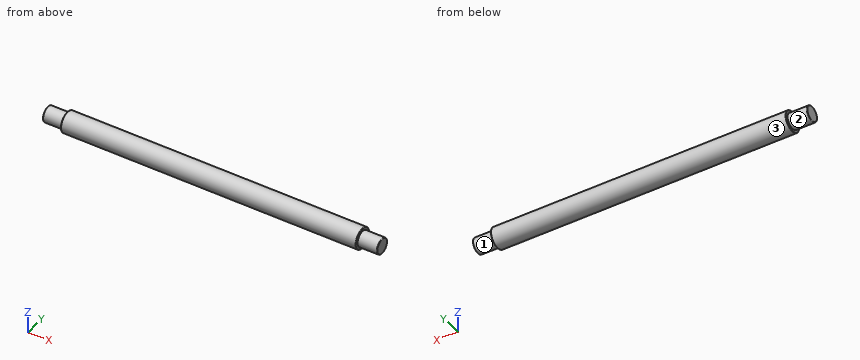
from build123d import *

# Parameters (mm, degrees)
RADYUS1_R = 1


with BuildPart() as part:
    # Çizim1 → Döndür1 (revolve)
    with BuildSketch(Plane.XY, mode=Mode.PRIVATE) as d_nd_r1_sk:
        Polygon((-324, 0), (-324, 15), (-286, 15), (-286, 20), (286, 20), (286, 15), (324, 15), (324, 0), align=None)
    revolve(d_nd_r1_sk.sketch.rotate(Axis((-324, 0, 0), (1, 0, 0)), 180), axis=Axis((-324, 0, 0), (1, 0, 0)))

    # Radyus1
    radyus1_edges = [part.edges().sort_by_distance(p)[0] for p in [
        (324, 15, 0),
        (286, 20, 0),
        (-286, 20, 0),
        (-324, 15, 0),
    ]]
    fillet(radyus1_edges, radius=RADYUS1_R)


solid = part.part
Read the model definition and answer for the solid it produces. Units are mm, in the model's axes. Face numbers are marked on the shaded views. A direction names the side the tool comes from. Round coordinates to 2 decimals unless told otherwise and drop trailing zeros. Order: outer loops, then holes, each group sorted by start corner. A loop starts at its lowest first (then second) coordinate and runs counter-clockwise, first axis right, second up. Notation, with made-up numbers: (23.25, -27) - (54.25, -27) arc R33 ccw to (54.25, 5) - close; hole circle Ø10 at (3.5, 13.5). An arc over 180 degrees is marked (long way). Use one line per item in the form item = value. Start each with the question number.
(1) Find the intervals of material crossed by line 1 along X through (y, z) = (17, -7); line 2 along Z through (x, y) = (53, 0); line 3 along Y through (x, z) = (-185, -1), in increasing order. Write a range as from..to.
(2) For the marked faces 1, 2 and 3, determine the directions among +Z, -Z, +X, -X, +Y, -Y from which every point of the face is accessible in a straight line to the end or side of a thin tool.
(3) The part is cut by section B-B (x = 16.5). Give the vertices of the cut face in (y, z).
(4) The part is cut by section A-A (y = 0). Give the vertices of the cut face in (x, z), then the cut area to 3 significant figures.
(5) Flat-ended cylindrical pins translate along their axes: pin 1 Ø1 at (x, y) = (-110, 14.5) entering from -Z; pin 2 Ø10 at (x, y) = (-173, 13.5) entering from +Z; pin 3 Ø12 at (x, z) = (235, -16) entering from +Y. Find the tip coordinate at first contact, or state that the pin passes through.
Checked values:
q1.line_1 = -286..286
q1.line_2 = -20..20
q1.line_3 = -19.97..19.97
q2.face_1 = +X
q2.face_2 = -X
q2.face_3 = +X, -X
q3.outline = circle Ø40 at (0, 0)
q4.outline = (-324, -14) arc R1 ccw to (-323, -15) - (-286, -15) - (-286, -19) arc R1 ccw to (-285, -20) - (285, -20) arc R1 ccw to (286, -19) - (286, -15) - (323, -15) arc R1 ccw to (324, -14) - (324, 14) arc R1 ccw to (323, 15) - (286, 15) - (286, 19) arc R1 ccw to (285, 20) - (-285, 20) arc R1 ccw to (-286, 19) - (-286, 15) - (-323, 15) arc R1 ccw to (-324, 14) - close
q4.area = 25,200 mm^2
q5.pin_1 = -14.28
q5.pin_2 = 18.1
q5.pin_3 = 17.32
